from build123d import *

# Parameters (mm, degrees)
BOSS_EXTRUDE1_DEPTH     = 50.8
F_1_4_CLEARANCE_HOLE1_D = 6.7564
F_1_4_CLEARANCE_HOLE2_D = 6.7564


with BuildPart() as part:
    # Sketch1 → Boss-Extrude1 (new body, symmetric)
    with BuildSketch(Plane.XY):
        with BuildLine():
            Line((-57.051702131, 6.35), (-70.104, 6.35))
            Line((-70.104, 6.35), (-70.104, 0))
            Line((-70.104, 0), (-51.203999954, 0))
            ThreePointArc((-51.203999954, 0), (-4.462722648, 51.009153275), (50.42609614, 8.891481281))
            Line((50.42609614, 8.891481281), (70.104, 8.891481281))
            Line((70.104, 8.891481281), (70.104, 15.241481281))
            Line((70.104, 15.241481281), (55.343621713, 15.241481281))
            ThreePointArc((55.343621713, 15.241481281), (-4.527029326, 57.22521491), (-57.051702131, 6.35))
        make_face()
    extrude(amount=BOSS_EXTRUDE1_DEPTH, both=True)

    # 1/4 Clearance Hole1 (through all)
    with Locations(Plane(origin=(0, 6.35, 0), x_dir=(1, 0, 0), z_dir=(0, 1, 0))):
        with Locations((-62.484, -31.75), (-62.484, 31.75)):
            Hole(F_1_4_CLEARANCE_HOLE1_D / 2)

    # 1/4 Clearance Hole2 (through all)
    with Locations(Plane(origin=(0, 15.241481281, 0), x_dir=(1, 0, 0), z_dir=(0, 1, 0))):
        with Locations((62.484, -31.75), (62.484, 31.75)):
            Hole(F_1_4_CLEARANCE_HOLE2_D / 2)


solid = part.part
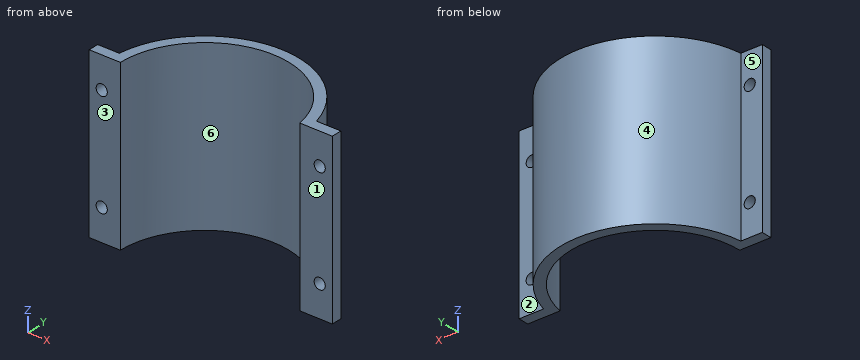
The listing builds one solid part. Answer for the finished solid, in the listing's coordinates (mm). Face numbers are marked on the shaded views. A direction names the side the tool comes from. Round coordinates to 2 decimals unless told otherwise and drop trailing zeros. Write each loop counter-clockwise with the first axis right and the second up, starting at its lowest first coordinate (ties: lowest second). Pieces come first, ordered by that corner, then holes. Notation, with made-up numbers: M 33.25,20.5 L 80.25,20.5 A13 ccw 80.25,36.5 Z; hole C 52,35 d1. An arc over 180 degrees is marked long. Write each question's results on one line, items separated by ' | '. Start each with the question number.
Item 1: Straight lines are drawn through the part: probe 1 along X at (y, z) = (13, -31); probe 2 along X at (y, z) = (11, 31.75); probe 3 along X at (y, z) = (6.5, 15.5). For each, find the intervals that lie inside material, in ascending order.
Item 2: Find section A-A on z = -31.75. Write down the section's boundary in (x, y), and give its area (3 significant figures).
Item 3: The mould has two halves that part along X. Classify the marked faces 4, 5 and 6: +X half, -X half, draft (parallel to the pull), parting line (faces both ways), or undercut.
Item 4: Find section C-C on y = 41. Write down the section's boundary in (x, z).
Item 5: Which of the six approach directions +Z, -Z, +X, -X, +Y, -Y give full straight-line access (tool end or side, diameter ignored) to the marked faces 1, 2 and 3?
Item 6: Given pin 1 Ø9 at (x, z) = (-62.484, 31.75) entering from +Y; pin 2 Ø3 at (y, z) = (47.5, 11) entering from +X; pin 3 Ø6 at (y, z) = (50.5, 14) entering from -X, each flat-ended and moving along its own axis, determine where each tip first touches the part or whether it passes through.
Item 7: Find section B-B on y = 17.5. Write down the section's boundary in (x, z).
Answer block:
1) probe 1: x = -55.91 to -49.53, 49.53 to 59.19, 65.78 to 70.1 | probe 2: x = -56.34 to -50.01, 50.01 to 59.11, 65.86 to 70.1 | probe 3: x = -57.03 to -50.79
2) outline: M -70.1,0 L -65.86,0 L -65.86,6.35 L -70.1,6.35 Z; M -59.11,0 L -51.2,0 A51.2 cw 50.43,8.89 L 59.11,8.89 L 59.11,15.24 L 55.34,15.24 A57.4 ccw -57.05,6.35 L -59.11,6.35 Z; M 65.86,8.89 L 70.1,8.89 L 70.1,15.24 L 65.86,15.24 Z | area: 1,090 mm²
3) face 4: parting line | face 5: draft | face 6: undercut
4) outline: M -40.18,-50.8 L -30.67,-50.8 L -30.67,50.8 L -40.18,50.8 Z; M 30.67,-50.8 L 40.18,-50.8 L 40.18,50.8 L 30.67,50.8 Z
5) face 1: +Z, -Z, +X, -Y | face 2: +Z, -Z, +X, +Y | face 3: +Z, -Z, +X, -X, -Y
6) pin 1: stops at y = 6.35 | pin 2: stops at x = 34.34 | pin 3: stops at x = -32.23
7) outline: M -54.67,-50.8 L -48.12,-50.8 L -48.12,50.8 L -54.67,50.8 Z; M 48.12,-50.8 L 54.67,-50.8 L 54.67,50.8 L 48.12,50.8 Z
